from build123d import *

# Parameters (mm, degrees)
SKETCH1_R           = 6.35
BOSS_EXTRUDE1_DEPTH = 9.525


with BuildPart() as part:
    # Sketch1 → Boss-Extrude1 (new body)
    with BuildSketch(Plane.XY):
        with BuildLine():
            Line((-25.4, 0), (-25.4, -6.052924625))
            Line((-25.4, -6.052924625), (17.310584604, -420.580806397))
            Line((17.310584604, -420.580806397), (-13.977037286, -420.580806397))
            Line((-13.977037286, -420.580806397), (-41.144220181, -33.731534677))
            Line((-41.144220181, -33.731534677), (-41.144220181, 0))
            ThreePointArc((-41.144220181, 0), (0, 41.144220181), (41.144220181, 0))
            Line((41.144220181, 0), (24.031627115, -8.224408685))
            ThreePointArc((24.031627115, -8.224408685), (25.055571523, -4.168733098), (25.4, 0))
            ThreePointArc((25.4, 0), (0, 25.4), (-25.4, 0))
        make_face()
        with Locations(Location((0, -406.4, 0), (0, 0, 180))):
            Circle(SKETCH1_R, mode=Mode.SUBTRACT)
    extrude(amount=BOSS_EXTRUDE1_DEPTH)


solid = part.part
Work out the finished part from the listing and answer in its coordinate system (mm). Give positions to 0.01 mm unless a question says otherwise; leave off trailing zeros. Loops run counter-clockwise (first coordinate to the right, second up) from the corner with the lowest first, then second, coordinate; pieces in that order, holes last. Notation, with made-up numbers: (-1.75, 46.25) -> (45.25, 46.25) arc R9 ccw to (45.25, 59.25) -> close; hole circle Ø1 at (48.25, 26). An arc over 180 degrees is marked (long way). Use a Markdown table: item, result. Add a question column.
1) The part is cut by section C-C, the plane x = 0. Determine the outline of the cut face in (y, z) (3 decimals).
2) Each of these flat-tipped pins is pushed along its axis until it touches: P1, Ø4, axis at y = -267, z = 3, coming from the -X side; P2, Ø1.8, axis at y = -3.5, z = 2.5, coming from the +X side. Where does it stop, or does it pass through?
3) The part is cut by section D-D, the plane y = -406.4. Determine the outline of the cut face in (x, z) (3 decimals), plus the area to 3 significant figures.
4) Consider line 1 along X through (y, z) = (-406.4, 2.5); line 2 along X through (y, z) = (22, 1.5); line 3 along X through (y, z) = (-276, 2). Determine where each line is inside the solid, lowest interval first.
5) The part is cut by section A-A, the plane z = 4.75. Determine the outline of the cut face in (x, y), plus the area to 3 significant figures.
6) For a pull along Y with two mould halves and no side action, classify faces 1 (the cylindrical face through (0.8, -412.7, 4.7)), 2 (the cylindrical face through (-0.905, 41.134, 4.696)), 3 (the flat face through (32.708, -4.055, 4.696)) as +Y half, -Y half, draft (parallel to the pull), parting line (faces both ways), or undercut.
7) The part is cut by section B-B, the plane y = 13. Determine the outline of the cut face in (x, z) (3 decimals).
Reported:
| question | item | result |
|---|---|---|
| 1 | outline | (-420.581, 0) -> (-412.75, 0) -> (-412.75, 9.525) -> (-420.581, 9.525) -> close; (-400.05, 0) -> (-252.573, 0) -> (-252.573, 9.525) -> (-400.05, 9.525) -> close; (25.4, 0) -> (41.144, 0) -> (41.144, 9.525) -> (25.4, 9.525) -> close |
| 2 | P1 | stops at x = -24.9 |
| 2 | P2 | stops at x = 35.73 |
| 3 | outline | (-14.973, 0) -> (-6.35, 0) -> (-6.35, 9.525) -> (-14.973, 9.525) -> close; (6.35, 0) -> (15.849, 0) -> (15.849, 9.525) -> (6.35, 9.525) -> close |
| 3 | area | 173 mm^2 |
| 4 | line 1 | x = -14.97 to -6.35, 6.35 to 15.85 |
| 4 | line 2 | x = -34.77 to -12.69, 12.69 to 34.77 |
| 4 | line 3 | x = -24.13 to 2.41 |
| 5 | outline | (-41.14, -33.73) -> (-13.98, -420.58) -> (17.31, -420.58) -> (-25.4, -6.05) -> (-25.4, 0) arc R25.4 cw (long way) to (24.03, -8.22) -> (41.14, 0) arc R41.14 ccw to (-41.14, 0) -> close; hole circle Ø12.7 at (0, -406.4) |
| 5 | area | 11,800 mm^2 |
| 6 | face 1 | undercut |
| 6 | face 2 | +Y half |
| 6 | face 3 | -Y half |
| 7 | outline | (-39.036, 0) -> (-21.821, 0) -> (-21.821, 9.525) -> (-39.036, 9.525) -> close; (21.821, 0) -> (39.036, 0) -> (39.036, 9.525) -> (21.821, 9.525) -> close |
